```python
from build123d import *

# Parameters (mm, degrees)
BOSS_EXTRUDE1_DEPTH       = 90
SHELL1_T                  = -2.5
FILLET1_R                 = 2.5
F_3_0MM_DOWEL_HOLE1_D     = 3
F_3_0MM_DOWEL_HOLE1_DEPTH = 2.5


with BuildPart() as part:
    # Sketch2 → Boss-Extrude1 (new body)
    with BuildSketch(Plane(origin=(0, 0, 0), x_dir=(0, 0, -1), z_dir=(1, 0, 0))):
        Polygon((0, 0), (80, 0), (80, 30), (0, 15), align=None)
    extrude(amount=BOSS_EXTRUDE1_DEPTH)

    # Shell1
    shell1_openings = [part.faces().sort_by_distance(p)[0] for p in [
        (45, 22.5, -40),
    ]]
    offset(amount=SHELL1_T, openings=shell1_openings, kind=Kind.INTERSECTION)

    # Fillet1
    fillet1_edges = [part.edges().sort_by_distance(p)[0] for p in [
        (90, 15, -80),
        (2.5, 8.984375, -2.5),
        (2.5, 2.5, -40),
        (45, 2.5, -2.5),
        (2.5, 16.015625, -77.5),
        (45, 2.5, -77.5),
        (87.5, 8.984375, -2.5),
        (87.5, 2.5, -40),
        (87.5, 16.015625, -77.5),
        (0, 15, -80),
        (45, 0, -80),
    ]]
    fillet(fillet1_edges, radius=FILLET1_R)

    # Ø3.0mm Dowel Hole1
    with Locations(Plane.XY):
        with Locations((25, 7.5), (65, 7.5)):
            Hole(F_3_0MM_DOWEL_HOLE1_D / 2, depth=F_3_0MM_DOWEL_HOLE1_DEPTH)


solid = part.part
```
Verification items for the finished model (mm, model axes). A direction names the side the tool comes from. Coordinates: 2 decimals unless noted, no trailing zeros. Loops run counter-clockwise (first coordinate to the right, second up) from the corner with the lowest first, then second, coordinate; pieces in that order, holes last. Notation, with made-up numbers: (37.5, 14) -> (69.5, 14) arc R22 cw to (69.5, 38) -> close; hole circle Ø9 at (79.25, 16). An arc over 180 degrees is marked (long way). Answer in a Markdown table with one row per item. Add a question column.
1. Section check D-D, the plane x = 38. Enter the section's corners in (y, z).
2. Access from +Z, -Z, +X, -X, +Y, -Y to the whole of each face (thin tool, end or side, straight path). Record for faces 4 (the face through (87.5, 15, -47)), 5 (the face through (45.63, 0.713, -79.248)), 6 (the face through (63.614, 6.925, -1.268)).
3. Section check A-A, the plane y = 7.5. Enter the section's corners in (x, z), then the cut area to 3 significant figures.
4. Material ranges on probe 1 along Z at (x, y) = (47, 11.25); probe 2 along X at (y, z) = (5, -40); probe 3 along Y at (x, z) = (41, -20), recorded low to high. Write a range as [from, to].
5. Depth check by flat-ended pin: P1, Ø1, axis at x = 16, y = 18, coming from the +Z side; P2, Ø2, axis at x = 52.5, z = -70.5, coming from the +Y side. Enter the tip coordinate at first touch or a pass-through.
6. Draft check along Y on faces 1 (the face through (26.2, 6.6, -1.3)), 2 (the face through (86.748, 3.213, -40.49)), 3 (the face through (3.252, 17.437, -76.787)). Enter one of: +Y half, -Y half, draft (parallel to the pull), parting line (faces both ways), or undercut.
7. Section check B-B, the plane x = 65. Enter the section's corners in (y, z), then the cut area to 3 significant figures.
8. Section check C-C, the plane y = 13.25. Enter the section's corners in (x, z).
Derived:
| question | item | result |
|---|---|---|
| 1 | outline | (0, -77.5) arc R2.5 ccw to (2.5, -80) -> (30, -80) -> (29.53, -77.5) -> (5, -77.5) arc R2.5 cw to (2.5, -75) -> (2.5, -5) arc R2.5 cw to (5, -2.5) -> (15.47, -2.5) -> (15, 0) -> (0, 0) -> close |
| 2 | face 4 | +Y |
| 2 | face 5 | -Z, +X, -X, -Y |
| 2 | face 6 | +Z |
| 3 | outline | (0, -77.5) arc R2.5 ccw to (2.5, -80) -> (87.5, -80) arc R2.5 ccw to (90, -77.5) -> (90, 0) -> (66.5, 0) -> (66.5, -2.5) -> (85, -2.5) arc R2.5 cw to (87.5, -5) -> (87.5, -75) arc R2.5 cw to (85, -77.5) -> (5, -77.5) arc R2.5 cw to (2.5, -75) -> (2.5, -5) arc R2.5 cw to (5, -2.5) -> (23.5, -2.5) -> (23.5, 0) -> (0, 0) -> close; (26.5, -2.5) -> (63.5, -2.5) -> (63.5, 0) -> (26.5, 0) -> close |
| 3 | area | 813 mm² |
| 4 | probe 1 | z = [-80, -77.5], [-2.5, 0] |
| 4 | probe 2 | x = [0, 2.5], [87.5, 90] |
| 4 | probe 3 | y = [0, 2.5] |
| 5 | P1 | stops at z = -77.5 |
| 5 | P2 | stops at y = 2.5 |
| 6 | face 1 | undercut |
| 6 | face 2 | +Y half |
| 6 | face 3 | draft |
| 7 | outline | (0, -77.5) arc R2.5 ccw to (2.5, -80) -> (30, -80) -> (29.53, -77.5) -> (5, -77.5) arc R2.5 cw to (2.5, -75) -> (2.5, -5) arc R2.5 cw to (5, -2.5) -> (6, -2.5) -> (6, 0) -> (0, 0) -> close; (9, -2.5) -> (15.47, -2.5) -> (15, 0) -> (9, 0) -> close |
| 7 | area | 294 mm² |
| 8 | outline | (0, -77.5) arc R2.5 ccw to (2.5, -80) -> (87.5, -80) arc R2.5 ccw to (90, -77.5) -> (90, 0) -> (0, 0) -> close; hole (2.5, -75) arc R2.5 ccw to (5, -77.5) -> (85, -77.5) arc R2.5 ccw to (87.5, -75) -> (87.5, -5) arc R2.5 ccw to (85, -2.5) -> (5, -2.5) arc R2.5 ccw to (2.5, -5) -> close |
